```python
from build123d import *

# Parameters (mm, degrees)
SKETCH1_W           = 120
SKETCH1_H           = 95
SKETCH1_W_2         = 310
SKETCH1_H_2         = 100
BOSS_EXTRUDE1_DEPTH = 5
SKETCH2_R           = 2
SKETCH2_W           = 25
SKETCH2_H           = 60
CUT_EXTRUDE1_DEPTH  = 6
FILLET1_R           = 5
SKETCH5_W           = 80
SKETCH5_H           = 70
CUT_EXTRUDE2_DEPTH  = 5
CHAMFER1_SIZE       = 20
SKETCH6_W           = 95
SKETCH6_H           = 95
BOSS_EXTRUDE2_DEPTH = 5
SKETCH7_W           = 310
SKETCH7_H           = 95
CUT_EXTRUDE3_DEPTH  = 6


with BuildPart() as part:
    # Sketch1 → Boss-Extrude1 (new body)
    with BuildSketch(Plane(origin=(0, 0, 0), x_dir=(1, 0, 0), z_dir=(0, 1, 0))):
        with Locations((0, 97.5)):
            Rectangle(SKETCH1_W, SKETCH1_H)
        Rectangle(SKETCH1_W_2, SKETCH1_H_2)
    extrude(amount=BOSS_EXTRUDE1_DEPTH)

    # Sketch2 → Cut-Extrude1 (cut, through all)
    with BuildSketch(Plane(origin=(0, 5, 0), x_dir=(1, 0, 0), z_dir=(0, 1, 0))):
        with Locations((-140, 40)):
            Circle(SKETCH2_R)
        with Locations((-125, 40)):
            Circle(SKETCH2_R)
        with Locations((-140, 25)):
            Circle(SKETCH2_R)
        with Locations((-140, 10)):
            Circle(SKETCH2_R)
        with Locations((140, 10)):
            Circle(SKETCH2_R)
        with Locations((140, 25)):
            Circle(SKETCH2_R)
        with Locations((125, 40)):
            Circle(SKETCH2_R)
        with Locations((140, 40)):
            Circle(SKETCH2_R)
        with Locations((-50, 130)):
            Circle(SKETCH2_R)
        with Locations((50, 130)):
            Circle(SKETCH2_R)
        Rectangle(SKETCH2_W, SKETCH2_H)
    extrude(amount=-CUT_EXTRUDE1_DEPTH, mode=Mode.SUBTRACT)

    # Fillet1
    fillet1_edges = [part.edges().sort_by_distance(p)[0] for p in [
        (12.5, 2.5, -30),
        (12.5, 2.5, 30),
        (-12.5, 2.5, 30),
        (-12.5, 2.5, -30),
    ]]
    fillet(fillet1_edges, radius=FILLET1_R)

    # Sketch5 → Cut-Extrude2 (cut)
    with BuildSketch(Plane(origin=(0, 5, 0), x_dir=(1, 0, 0), z_dir=(0, 1, 0))):
        with Locations((0, 85)):
            Rectangle(SKETCH5_W, SKETCH5_H)
    extrude(amount=-CUT_EXTRUDE2_DEPTH, mode=Mode.SUBTRACT)

    # Chamfer1
    chamfer1_edges = [part.edges().sort_by_distance(p)[0] for p in [
        (40, 2.5, -50),
        (-40, 2.5, -50),
        (-40, 2.5, -120),
        (40, 2.5, -120),
    ]]
    chamfer(chamfer1_edges, length=CHAMFER1_SIZE)

    # Sketch6 → Boss-Extrude2 (add)
    with BuildSketch(Plane(origin=(0, 5, 0), x_dir=(1, 0, 0), z_dir=(0, 1, 0))):
        with Locations((107.5, 97.5)):
            Rectangle(SKETCH6_W, SKETCH6_H)
        with Locations((-107.5, 97.5)):
            Rectangle(SKETCH6_W, SKETCH6_H)
    extrude(amount=-BOSS_EXTRUDE2_DEPTH)

    # Sketch7 → Cut-Extrude3 (cut, through all)
    with BuildSketch(Plane(origin=(0, 5, 0), x_dir=(1, 0, 0), z_dir=(0, 1, 0))):
        with Locations((0, 97.5)):
            Rectangle(SKETCH7_W, SKETCH7_H)
    extrude(amount=-CUT_EXTRUDE3_DEPTH, mode=Mode.SUBTRACT)


solid = part.part
```
Geometry: final body of the model. Coordinates: model frame, mm. A direction names the side the tool comes from. Coordinates: 2 decimals unless noted, no trailing zeros. Order: outer loops, then holes, each group sorted by start corner. A loop starts at its lowest first (then second) coordinate and runs counter-clockwise, first axis right, second up. Notation, with made-up numbers: M -39.5,31 L -21.5,31 A18 cw -21.5,61 Z; hole C 18.25,34.25 d5. An arc over 180 degrees is marked long. Answer in a Markdown table with one row per item. Add a question column.
Q1. Section query A-A on z = -3. Return the cut outline in (x, y).
Q2. Mould query, pull axis Z, two halves, no side actions, for faces 3 (the flat face through (-2, 3, -50)), 4 (the flat face through (0, 3, -30)), 5 (the flat face through (32, 5, -1)), 6 (the cylindrical face through (11, 2.46, 28.57)). Classes: released by +Z, released by -Z, zero draft, split by the parting line, or undercut.
Q3. Line query: L1, parallel to Z at x = -140, y = 2.7; L2, parallel to X at y = 2.7, z = -25; L3, parallel to X at y = 2.3, z = -4. Output: solid intervals per line, ascending.
Q4. Section query B-B on y = 1.6. Count the separate pieces of the cut face and the enclosed holes in it, and give its area (3 significant figures).
Q5. Reachability of faces 1 (the flat face through (155, 3, 1)), 2 (the flat face through (12.5, 3, 0)) from +Z, -Z, +X, -X, +Y, -Y: full face, straight path, thin tool, end or side. Return the list, or none.
Completed:
| question | item | result |
|---|---|---|
| 1 | outline | M -155,0 L -12.5,0 L -12.5,5 L -155,5 Z; M 12.5,0 L 155,0 L 155,5 L 12.5,5 Z |
| 2 | face 3 | released by -Z |
| 2 | face 4 | undercut |
| 2 | face 5 | zero draft |
| 2 | face 6 | undercut |
| 3 | L1 | z = -50 to -42, -38 to -27, -23 to -12, -8 to 50 |
| 3 | L2 | x = -155 to -142, -138 to -12.5, 12.5 to 138, 142 to 155 |
| 3 | L3 | x = -155 to -12.5, 12.5 to 155 |
| 4 | separate pieces | 1 |
| 4 | enclosed holes | 9 |
| 4 | area | 29,400 mm2 |
| 5 | face 1 | +Z, -Z, +X, +Y, -Y |
| 5 | face 2 | +Y, -Y |
